For this review, take the finished solid that the model builds, in its own axes (mm). A direction names the side the tool comes from. Round coordinates to 2 decimals unless told otherwise and drop trailing zeros. Write each loop counter-clockwise with the first axis right and the second up, starting at its lowest first coordinate (ties: lowest second). Pieces come first, ordered by that corner, then holes. Notation, with made-up numbers: (46.25, -1.75) - (71.25, -1.75) arc R17 ccw to (71.25, 6.25) - close; hole circle Ø7 at (-24.75, 85.5). An arc over 180 degrees is marked (long way). Answer in a Markdown table with one row per item. Add a question column.
from build123d import *

# Parameters (mm, degrees)
SKETCH1_W                  = 16
SKETCH1_H                  = 6.5
BOSS_EXTRUDE1_DEPTH        = 4
SKETCH2_W                  = 8
SKETCH2_H                  = 6.5
CUT_EXTRUDE1_DEPTH         = 6.5
SKETCH10_W                 = 4
SKETCH10_H                 = 4
BOSS_EXTRUDE2_DEPTH        = 3
M1_6_CLEARANCE_HOLE1_D     = 2
M1_6_CLEARANCE_HOLE1_DEPTH = 4
M1_6_CLEARANCE_HOLE1_TIP   = 0.600860619
FILLET1_R                  = 1
FILLET2_R                  = 2.5
SKETCH14_W                 = 3.5
SKETCH14_H                 = 4.5
CUT_EXTRUDE3_DEPTH         = 5
M2_CLEARANCE_HOLE3_D       = 2.6
M2_CLEARANCE_HOLE3_DEPTH   = 4
M2_CLEARANCE_HOLE3_TIP     = 0.781118805


with BuildPart() as part:
    # Sketch1 → Boss-Extrude1 (new body, symmetric)
    with BuildSketch(Plane(origin=(0, 0, 0), x_dir=(1, 0, 0), z_dir=(0, 1, 0))):
        Rectangle(SKETCH1_W, SKETCH1_H)
    extrude(amount=BOSS_EXTRUDE1_DEPTH, both=True)

    # Sketch2 → Cut-Extrude1 (cut)
    with BuildSketch(Plane(origin=(0, 4, 5), x_dir=(1, 0, 0), z_dir=(0, -1, 0))):
        with Locations((0, -5)):
            Rectangle(SKETCH2_W, SKETCH2_H)
    extrude(amount=CUT_EXTRUDE1_DEPTH, mode=Mode.SUBTRACT)

    # Sketch10 → Boss-Extrude2 (add)
    with BuildSketch(Plane.XZ.offset(4)):
        with Locations((6, -5.25)):
            Rectangle(SKETCH10_W, SKETCH10_H)
        with Locations((-6, -5.25)):
            Rectangle(SKETCH10_W, SKETCH10_H)
    extrude(amount=-BOSS_EXTRUDE2_DEPTH)

    # M1.6 Clearance Hole1
    with Locations(Plane(origin=(0, -1, 0), x_dir=(1, 0, 0), z_dir=(0, 1, 0))):
        with Locations((6, 5.25), (-6, 5.25)):
            Hole(M1_6_CLEARANCE_HOLE1_D / 2, depth=M1_6_CLEARANCE_HOLE1_DEPTH)
            with Locations((0, 0, -(M1_6_CLEARANCE_HOLE1_DEPTH + M1_6_CLEARANCE_HOLE1_TIP / 2))):  # 118° drill point
                Cone(0, M1_6_CLEARANCE_HOLE1_D / 2, M1_6_CLEARANCE_HOLE1_TIP, mode=Mode.SUBTRACT)

    # Fillet1
    fillet1_edges = [part.edges().sort_by_distance(p)[0] for p in [
        (4, -2.5, 0),
        (-4, -2.5, 0),
    ]]
    fillet(fillet1_edges, radius=FILLET1_R)

    # Fillet2
    fillet2_edges = [part.edges().sort_by_distance(p)[0] for p in [
        (-4, -3.25, -3.25),
        (4, -3.25, -3.25),
    ]]
    fillet(fillet2_edges, radius=FILLET2_R)

    # Sketch14 → Cut-Extrude3 (cut)
    with BuildSketch(Plane(origin=(8, 0, 0), x_dir=(0, 0, -1), z_dir=(1, 0, 0))):
        with Locations((-1.5, 0.25)):
            Rectangle(SKETCH14_W, SKETCH14_H)
    extrude(amount=-CUT_EXTRUDE3_DEPTH, mode=Mode.SUBTRACT)

    # M2 Clearance Hole3
    with Locations(Plane.ZY.offset(8)):
        with Locations((1.5, 0.25)):
            Hole(M2_CLEARANCE_HOLE3_D / 2, depth=M2_CLEARANCE_HOLE3_DEPTH)
            with Locations((0, 0, -(M2_CLEARANCE_HOLE3_DEPTH + M2_CLEARANCE_HOLE3_TIP / 2))):  # 118° drill point
                Cone(0, M2_CLEARANCE_HOLE3_D / 2, M2_CLEARANCE_HOLE3_TIP, mode=Mode.SUBTRACT)


solid = part.part
Q1. Insertion check: pin 1 Ø3 at (x, y) = (5.5, 1.5) entering from -Z; pin 2 Ø1.8 at (x, z) = (1, 0) entering from +Y; pin 3 Ø4.5 at (x, z) = (-6, -6) entering from +Y. Each pin has a flat end and moves straight along its axis. Give the tip position at first contact, or say it passes through.
Q2. To check wall thickness, follow probe 1 along Z at (x, y) = (6, -3.2); probe 2 along X at (y, z) = (-2.8, -5.25); probe 3 along X at (y, z) = (1.5, -2.5). State the ranges of each line that lie inside material, in increasing order.
Q3. Add section A-A on x = -6. State the section outline as (y, z) points, then the cut area to 3 significant figures.
Q4. Add section B-B on y = 0.25. State the section outline as (x, z) points, then the cut area to 3 significant figures.
Q5. Tool access review of faces 4 (the face through (6, -2, 2)), 5 (the face through (3.715, -2.199, -1.187)), 6 (the face through (-3.564, -3.01, -4.339)), 7 (the face through (6, 2, -3.25)): name each direction out of +Z, -Z, +X, -X, +Y, -Y from which nothing blocks a thin tool from reaching the whole face with its end or side.
Q6. Add section D-D on z = 1.5. State the section outline as (x, y) points, then the cut area to 3 significant figures.
Q7. Add section C-C on x = 6. State the section outline as (y, z) points.
Q8. Draft analysis for pull direction Z (two halves, no side actions). For faces 1 (the face through (6, 0, -0.25)), 2 (the face through (0, -3, -3.25)), 3 (the face through (-6, 0.3, 2.8)), state which applies: released by +Z, released by -Z, zero draft, split by the parting line, or undercut.
Answer sheet:
| question | item | result |
|---|---|---|
| 1 | pin 1 | stops at z = -3.25 |
| 1 | pin 2 | stops at y = -2.5 |
| 1 | pin 3 | stops at y = -1 |
| 2 | probe 1 | z = -7.25 to -6.25, -4.25 to 3.25 |
| 2 | probe 2 | x = -8 to -7, -5 to -3.95, 3.95 to 5, 7 to 8 |
| 2 | probe 3 | x = -8 to -4, 4 to 8 |
| 3 | outline | (-4, -7.25) - (-1, -7.25) - (-1, -6.25) - (-4, -6.25) - close; (-4, -4.25) - (-1, -4.25) - (-1, -3.25) - (4, -3.25) - (4, 3.25) - (-4, 3.25) - close; hole circle Ø2.6 at (0.25, 1.5) |
| 3 | area | 52.7 mm² |
| 4 | outline | (-8, -3.25) - (-4, -3.25) - (-4, 0.2) - (-8, 0.2) - close; (-8, 2.8) - (-4, 2.8) - (-4, 3.25) - (-8, 3.25) - close; (4, -3.25) - (8, -3.25) - (8, -0.25) - (4, -0.25) - close |
| 4 | area | 27.6 mm² |
| 5 | face 4 | +Z, +X |
| 5 | face 5 | +Z, -Z, +Y |
| 5 | face 6 | -Z, +Y, -Y |
| 5 | face 7 | -Z, +X, -X, +Y |
| 6 | outline | (-8, -4) - (8, -4) - (8, -2) - (3.87, -2) arc R1 cw to (3, -2.5) - (-3, -2.5) arc R1 cw to (-4, -1.5) - (-4, -1.05) - (-8, -1.05) - close; (-8, 1.55) - (-4, 1.55) - (-4, 4) - (-8, 4) - close; (4, 2.5) - (8, 2.5) - (8, 4) - (4, 4) - close |
| 6 | area | 48.0 mm² |
| 7 | outline | (-4, -7.25) - (-1, -7.25) - (-1, -6.25) - (-4, -6.25) - close; (-4, -4.25) - (-1, -4.25) - (-1, -3.25) - (4, -3.25) - (4, 3.25) - (2.5, 3.25) - (2.5, -0.25) - (-2, -0.25) - (-2, 3.25) - (-4, 3.25) - close |
| 8 | face 1 | released by +Z |
| 8 | face 2 | released by -Z |
| 8 | face 3 | undercut |
